Geometry check sheet. Reference: the model listing, model coordinates, mm. Face numbers are marked on the shaded views. A direction names the side the tool comes from. Round coordinates to 2 decimals unless told otherwise and drop trailing zeros. Order: outer loops, then holes, each group sorted by start corner. A loop starts at its lowest first (then second) coordinate and runs counter-clockwise, first axis right, second up. Notation, with made-up numbers: (26.5, 68.5) - (56.5, 68.5) arc R16 cw to (56.5, 84.5) - close; hole circle Ø7 at (74, 55). An arc over 180 degrees is marked (long way). Write each question's results on one line, items separated by ' | '.
```python
from build123d import *

# Parameters (mm, degrees)
SKETCH001_W  = 2
SKETCH001_H  = 16
POCKET_DEPTH = 1.9


with BuildPart() as part:
    # Sketch → Revolution (revolve)
    with BuildSketch(Plane.YZ):
        Polygon((0, 0), (0, 7), (1, 8), (3.8, 8), (3.8, 5), (13.8, 5), (13.8, 3.235), (17.758327, 3.235), (18.2, 4), (24.358327, 4), (24.8, 3.235), (24.8, 0), align=None)
    revolve(axis=Axis((0, 0, 0), (0, 1, 0)))

    # Sketch001 → Pocket (cut)
    with BuildSketch(Plane(origin=(0, 0, 0), x_dir=(0, 0, -1), z_dir=(0, -1, 0))):
        Rectangle(SKETCH001_W, SKETCH001_H)
    extrude(amount=-POCKET_DEPTH, mode=Mode.SUBTRACT)


solid = part.part
```
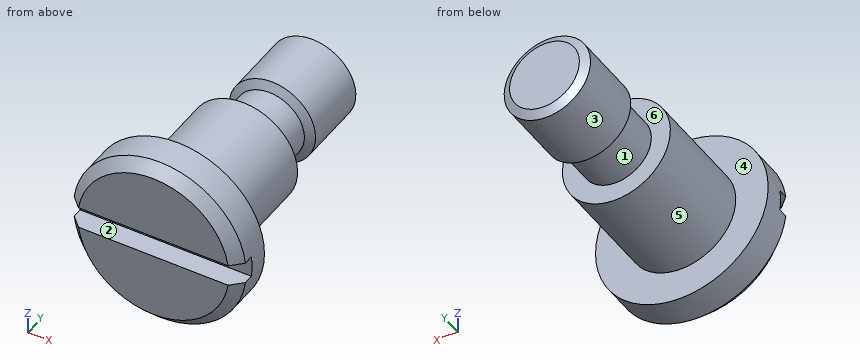
(1) Depth check by flat-ended pin: pin 1 Ø1 at (x, y) = (1, 1) entering from -Z; pin 2 Ø8 at (x, y) = (5.5, 11) entering from +Z; pin 3 Ø1.6 at (x, z) = (-0.5, 0) entering from -Y. Enter the tip coordinate at first touch or a pass-through.
Answers follow:
pin 1: z = -7.98 | pin 2: z = 4.77 | pin 3: y = 1.9
(2) Draft check along Y on the marked faces 4, 5 and 6. Enter one of: released by +Y, released by -Y, zero draft, split by the parting line, or undercut.
Answers follow:
face 4: released by +Y | face 5: zero draft | face 6: undercut
(3) Section check D-D (y = 16.5). Record the cut outline in (x, z) (3 decimals), then the cut area to 3 significant figures.
Answers follow:
outline: circle Ø6.47 at (0, 0) | area: 32.9 mm²
(4) Material ranges on line 1 (Y direction, x = -2.75, z = 4.75); line 2 (Y direction, x = -4.75, z = -0.5); line 3 (Z direction, x = -1.25, y = 1.5), recorded low to high.
Answers follow:
line 1: 0 to 3.8 | line 2: 1.9 to 13.8 | line 3: -7.9 to -1, 1 to 7.9
(5) Section check A-A (x = 0). Record the cut outline in (y, z) (3 decimals), then the cut area to 3 significant figures.
Answers follow:
outline: (0, -7) - (1, -8) - (3.8, -8) - (3.8, -5) - (13.8, -5) - (13.8, -3.235) - (17.758, -3.235) - (18.2, -4) - (24.358, -4) - (24.8, -3.235) - (24.8, 3.235) - (24.358, 4) - (18.2, 4) - (17.758, 3.235) - (13.8, 3.235) - (13.8, 5) - (3.8, 5) - (3.8, 8) - (1, 8) - (0, 7) - (0, 1) - (1.9, 1) - (1.9, -1) - (0, -1) - close | area: 237 mm²
(6) Section check C-C (y = 6.5). Record the cut outline in (x, z).
Answers follow:
outline: circle Ø10 at (0, 0)
(7) Access from +Z, -Z, +X, -X, +Y, -Y to the whole of each face (thin tool, end or side, straight path). Record for the marked faces 1, 2 and 3.
Answers follow:
face 1: none | face 2: +X, -X, -Y | face 3: +Y
(8) Section check B-B (z = 0). Record the cut outline in (x, y) (3 decimals).
Answers follow:
outline: (-8, 1.9) - (8, 1.9) - (8, 3.8) - (5, 3.8) - (5, 13.8) - (3.235, 13.8) - (3.235, 17.758) - (4, 18.2) - (4, 24.358) - (3.235, 24.8) - (-3.235, 24.8) - (-4, 24.358) - (-4, 18.2) - (-3.235, 17.758) - (-3.235, 13.8) - (-5, 13.8) - (-5, 3.8) - (-8, 3.8) - close
